Here's how the part is built. I have some questions about the finished solid (model axes, mm). Coordinates: 2 decimals unless noted, no trailing zeros. Loops run counter-clockwise (first coordinate to the right, second up) from the corner with the lowest first, then second, coordinate; pieces in that order, holes last. Notation, with made-up numbers: (51.5, -25) -> (63.5, -25) arc R15 cw to (63.5, -7) -> close; hole circle Ø4 at (28.25, 54.5). An arc over 180 degrees is marked (long way). Answer as a JSON object with one key per item and string values. Group by question number.
1) I want a section at A-A (x = 75.5). Write out the boundary of the cut face in (y, z) (3 decimals).
2) I'm going to push a flat-ended pin straight in: pin 1 (3 mm diameter, centred on x = 184.5, y = -3.5, fed in from +Z). Where does the tip first touch, or does it pass through?
3) I need wall thicknesses on probe 1 along Y at (x, z) = (296, -0.5); probe 2 along Z at (x, y) = (219.5, 0); probe 3 along Y at (x, z) = (257.5, 0). Which ranges of each line are inside material? Lowest first, please. Write a range as [from, to].
```python
from build123d import *

# Parameters (mm, degrees)
SKETCH1_R           = 2.0193
BOSS_EXTRUDE1_DEPTH = 714.375
SKETCH2_R           = 1.524
CUT_EXTRUDE1_DEPTH  = 715.440848817
SKETCH3_R           = 21.255995951
CUT_EXTRUDE2_DEPTH  = 6.35


with BuildPart() as part:
    # Sketch1 → Boss-Extrude1 (new body)
    with BuildSketch(Plane(origin=(0, 0, 0), x_dir=(0, 0, -1), z_dir=(1, 0, 0))):
        Polygon((7.332348419, 0), (3.666174209, 6.35), (-3.666174209, 6.35), (-7.332348419, 0), (-3.666174209, -6.35), (3.666174209, -6.35), align=None)
        Circle(SKETCH1_R, mode=Mode.SUBTRACT)
    extrude(amount=BOSS_EXTRUDE1_DEPTH)

    # Sketch2 → Cut-Extrude1 (cut, through all)
    with BuildSketch(Plane(origin=(714.375, 0, 0), x_dir=(0, 0, -1), z_dir=(1, 0, 0))):
        with Locations((0, 6.35)):
            Circle(SKETCH2_R)
        with Locations((5.499261314, 3.175)):
            Circle(SKETCH2_R)
        with Locations((5.499261314, -3.175)):
            Circle(SKETCH2_R)
        with Locations((0, -6.35)):
            Circle(SKETCH2_R)
        with Locations((-5.499261314, -3.175)):
            Circle(SKETCH2_R)
        with Locations((-5.499261314, 3.175)):
            Circle(SKETCH2_R)
    extrude(amount=-CUT_EXTRUDE1_DEPTH, mode=Mode.SUBTRACT)

    # Sketch3 → Cut-Extrude2 (cut)
    with BuildSketch(Plane(origin=(714.375, 0, 0), x_dir=(0, 0, -1), z_dir=(1, 0, 0))):
        Circle(SKETCH3_R)
    extrude(amount=-CUT_EXTRUDE2_DEPTH, mode=Mode.SUBTRACT)


solid = part.part
```
Determined:
{
 "1": {"outline": "(-6.35, -3.666) -> (-4.495, -4.737) arc R1.524 cw to (-1.855, -6.261) -> (0, -7.332) -> (1.855, -6.261) arc R1.524 cw to (4.495, -4.737) -> (6.35, -3.666) -> (6.35, -1.524) arc R1.524 cw to (6.35, 1.524) -> (6.35, 3.666) -> (4.495, 4.737) arc R1.524 cw to (1.855, 6.261) -> (0, 7.332) -> (-1.855, 6.261) arc R1.524 cw to (-4.495, 4.737) -> (-6.35, 3.666) -> (-6.35, 1.524) arc R1.524 cw to (-6.35, -1.524) -> close; hole circle Ø4.039 at (0, 0)"},
 "2": {"pin 1": "z = 4.74"},
 "3": {"probe 1": "[-4.91, -1.96], [1.96, 4.91]", "probe 2": "[-7.33, -2.02], [2.02, 7.33]", "probe 3": "[-4.83, -2.02], [2.02, 4.83]"}
}
